Geometry check sheet. Reference: the model listing, model coordinates, mm. A direction names the side the tool comes from. Round coordinates to 2 decimals unless told otherwise and drop trailing zeros. Order: outer loops, then holes, each group sorted by start corner. A loop starts at its lowest first (then second) coordinate and runs counter-clockwise, first axis right, second up. Notation, with made-up numbers: (65, 54) -> (93, 54) arc R32 ccw to (93, 87) -> close; hole circle Ø4 at (17.25, -35). An arc over 180 degrees is marked (long way). Use a Markdown table: item, result. Add a question column.
Item 1: Set-up check for faces 4 (the flat face through (-8, 0, -6)), 5 (the cylindrical face through (25, 7, 22)): record each of +Z, -Z, +X, -X, +Y, -Y from which the full face is reachable in a straight line by a thin tool's end or side.
Item 2: Mould release check, pull along X, two halves, no side actions. Record for faces 1 (the flat face through (-8, 10, -6)), 2 (the cylindrical face through (-15.89, 4.93, -13.257)), 3 (the flat face through (-35, 5, 0)): pulls with the +X half, pulls with the -X half, needs draft (parallel to the pull), parting line crosses it, or undercut.
Item 3: Sectioned sample at D-D, the plane z = -0.5. Record the cut outline in (x, y), and give its area (3 significant figures).
Item 4: Sectioned sample at C-C, the plane y = 2. Record the cut outline in (x, z).
Item 5: Sectioned sample at A-A, the plane x = -25. Record the cut outline in (y, z).
Item 6: Sectioned sample at B-B, the plane z = 15. Record the cut outline in (x, y).
Item 7: Gauge pin test, flat end, axial feed: pin 1 Ø3 at (x, y) = (-25, 5) entering from +Z. Record the tip position at first contact, or that the pin passes through.
Item 8: Material ranges on probe 1 along Z at (x, y) = (-15.5, 7.5); probe 2 along X at (y, z) = (5, 23); probe 3 along Z at (x, y) = (0, 2.75), recorded low to high. Write a range as [from, to].
from build123d import *

# Parameters (mm, degrees)
SKETCH2_W           = 70
SKETCH2_H           = 50
BOSS_EXTRUDE1_DEPTH = 10
SKETCH3_R           = 4
CUT_EXTRUDE1_DEPTH  = 11
SKETCH4_R           = 1.8
CUT_EXTRUDE2_DEPTH  = 11
SKETCH5_R           = 10
CUT_EXTRUDE3_DEPTH  = 11
SKETCH6_R           = 2
CUT_EXTRUDE5_DEPTH  = 10


with BuildPart() as part:
    # Sketch2 → Boss-Extrude1 (new body)
    with BuildSketch(Plane(origin=(0, 0, 0), x_dir=(1, 0, 0), z_dir=(0, 1, 0))):
        Rectangle(SKETCH2_W, SKETCH2_H)
    extrude(amount=BOSS_EXTRUDE1_DEPTH)

    # Sketch3 → Cut-Extrude1 (cut, through all)
    with BuildSketch(Plane(origin=(0, 10, 0), x_dir=(1, 0, 0), z_dir=(0, 1, 0))):
        with Locations((-25, -15)):
            Circle(SKETCH3_R)
        with Locations((25, -15)):
            Circle(SKETCH3_R)
    extrude(amount=-CUT_EXTRUDE1_DEPTH, mode=Mode.SUBTRACT)

    # Sketch4 → Cut-Extrude2 (cut, through all)
    with BuildSketch(Plane.XZ):
        with Locations((-15.5, 19.5)):
            Circle(SKETCH4_R)
        with Locations((-15.5, -11.5)):
            Circle(SKETCH4_R)
        with Locations((15.5, -11.5)):
            Circle(SKETCH4_R)
        with Locations((15.5, 19.5)):
            Circle(SKETCH4_R)
    extrude(amount=-CUT_EXTRUDE2_DEPTH, mode=Mode.SUBTRACT)

    # Sketch5 → Cut-Extrude3 (cut, through all)
    with BuildSketch(Plane.XZ):
        with Locations((0, 4)):
            Circle(SKETCH5_R)
    extrude(amount=-CUT_EXTRUDE3_DEPTH, mode=Mode.SUBTRACT)

    # Sketch6 → Cut-Extrude5 (cut)
    with BuildSketch(Plane.XY.offset(25)):
        with Locations((25, 5)):
            Circle(SKETCH6_R)
        with Locations((-25, 5)):
            Circle(SKETCH6_R)
    extrude(amount=-CUT_EXTRUDE5_DEPTH, mode=Mode.SUBTRACT)


solid = part.part
Found:
| question | item | result |
|---|---|---|
| 1 | face 4 | +Z, -Z, +X, -X, -Y |
| 1 | face 5 | +Z |
| 2 | face 1 | needs draft |
| 2 | face 2 | undercut |
| 2 | face 3 | pulls with the -X half |
| 3 | outline | (-35, 0) -> (-8.93, 0) -> (-8.93, 10) -> (-35, 10) -> close; (8.93, 0) -> (35, 0) -> (35, 10) -> (8.93, 10) -> close |
| 3 | area | 521 mm2 |
| 4 | outline | (-35, -25) -> (35, -25) -> (35, 25) -> (-35, 25) -> close; hole circle Ø8 at (-25, 15); hole circle Ø3.6 at (-15.5, -11.5); hole circle Ø3.6 at (-15.5, 19.5); hole circle Ø20 at (0, 4); hole circle Ø3.6 at (15.5, -11.5); hole circle Ø3.6 at (15.5, 19.5); hole circle Ø8 at (25, 15) |
| 5 | outline | (0, -25) -> (10, -25) -> (10, 11) -> (0, 11) -> close; (0, 19) -> (3, 19) -> (3, 25) -> (0, 25) -> close; (7, 19) -> (10, 19) -> (10, 25) -> (7, 25) -> close |
| 6 | outline | (-35, 0) -> (-29, 0) -> (-29, 10) -> (-35, 10) -> close; (-21, 0) -> (21, 0) -> (21, 10) -> (-21, 10) -> close; (29, 0) -> (35, 0) -> (35, 10) -> (29, 10) -> close |
| 7 | pin 1 | stops at z = 11.29 |
| 8 | probe 1 | z = [-25, -13.3], [-9.7, 17.7], [21.3, 25] |
| 8 | probe 2 | x = [-35, -27], [-23, 23], [27, 35] |
| 8 | probe 3 | z = [-25, -6], [14, 25] |
